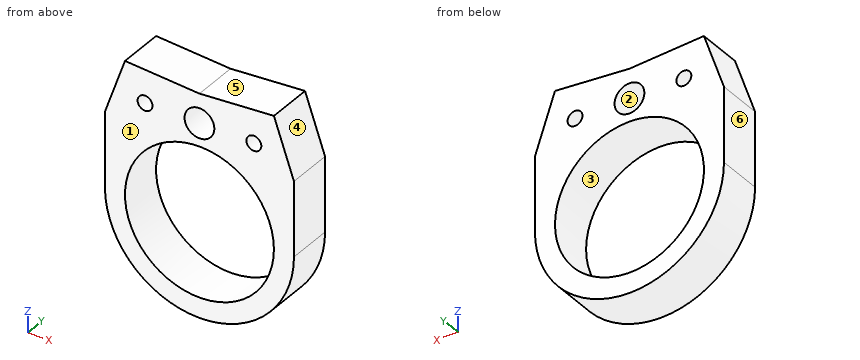
from build123d import *

# Parameters (mm, degrees)
F0_R     = 8.255
F1_DEPTH = 5.08
F3_DEPTH = 5.08
F4_R     = 1.651
F4_R_2   = 0.8255
F5_DEPTH = 25.4


with BuildPart() as f1:
    # F0 (on Front) → F1 (new body)
    with BuildSketch(Plane.XZ):
        with BuildLine():
            ThreePointArc((-10.4775, 0), (0, 10.4775), (10.4775, 0))
            Line((10.4775, 0), (10.4775, 8.255))
            Line((10.4775, 8.255), (6.0325, 10.795))
            Line((6.0325, 10.795), (-6.0325, 10.795))
            Line((-6.0325, 10.795), (-10.4775, 8.255))
            Line((-10.4775, 8.255), (-10.4775, 0))
        make_face()
        with BuildLine():
            ThreePointArc((-10.4775, 0), (0, -10.4775), (10.4775, 0))
            ThreePointArc((10.4775, 0), (0, 10.4775), (-10.4775, 0))
        make_face()
        Circle(F0_R, mode=Mode.SUBTRACT)
    extrude(amount=F1_DEPTH)

    # F2 (on face) → F3 (join)
    with BuildSketch(Plane.XZ.offset(5.08)):
        Polygon((0, 14.0335), (-8.255, 14.605), (-10.4775, 8.255), (-6.0325, 10.795), (6.0325, 10.795), (10.4775, 8.255), (8.255, 14.605), align=None)
    extrude(amount=-F3_DEPTH)

    # F4 (on face) → F5 (cut)
    with BuildSketch(Plane.XZ.offset(5.08)):
        with Locations((0, 10.795)):
            Circle(F4_R)
        with Locations((6.0325, 10.795)):
            Circle(F4_R_2)
        with Locations((-6.0325, 10.795)):
            Circle(F4_R_2)
    extrude(amount=-F5_DEPTH, mode=Mode.SUBTRACT)


solid = f1.part
Work out the finished part from the listing and answer in its coordinate system (mm). Face numbers are marked on the shaded views. A direction names the side the tool comes from. Give positions to 0.01 mm unless a question says otherwise; leave off trailing zeros. Write each loop counter-clockwise with the first axis right and the second up, starting at its lowest first coordinate (ties: lowest second). Pieces come first, ordered by that corner, then holes.
Q1. Given pin 1 (2 mm diameter, centred on y = -1, z = -3, fed in from -X); pin 2 (1.3 mm diameter, centred on x = -6.03, z = 10.8, fed in from -Y); pin 3 (1.5 mm diameter, centred on y = -4, z = -2, fed in from -X), each flat-ended and moving along its own axis, determine where each tip first touches the part or whether it passes through.
Answer:
pin 1: stops at x = -10.28
pin 2: passes through
pin 3: stops at x = -10.4
Q2. The part is cut by section B-B on x = -2. Give the vertices of the cut face in (y, z).
Answer:
outline: (-5.08, -10.28) - (0, -10.28) - (0, -8.01) - (-5.08, -8.01) - close; (-5.08, 8.01) - (0, 8.01) - (0, 14.17) - (-5.08, 14.17) - close
Q3. The part is cut by section A-A on z = -7. Give the vertices of the cut face in (x, y), and give its area (3 significant figures).
Answer:
outline: (-7.8, -5.08) - (-4.38, -5.08) - (-4.38, 0) - (-7.8, 0) - close; (4.38, -5.08) - (7.8, -5.08) - (7.8, 0) - (4.38, 0) - close
area: 34.8 mm2
Q4. Straight lines are drawn through the part: L1, parallel to Z at x = 0, y = -1.9 (1 decimal); L2, parallel to Z at x = -6, y = -1.5; L3, parallel to X at y = -0.25, z = -2.75. For each, find the intervals that lie inside material, in ascending order.
Answer:
L1: z = -10.5 to -8.3, 8.3 to 9.1, 12.4 to 14
L2: z = -8.59 to -5.67, 5.67 to 9.97, 11.62 to 14.45
L3: x = -10.11 to -7.78, 7.78 to 10.11
Q5. For a pull along X with two mould halves and no side action, classify the marked faces 1, 2, 3 and 4 as released by +X, released by -X, zero draft, split by the parting line, or undercut.
Answer:
face 1: zero draft
face 2: undercut
face 3: undercut
face 4: released by +X
Q6. The part is cut by section C-C on y = -2.75. Give the vertices of the cut face in (x, z) (1 decimal).
Answer:
outline: (-10.5, 0) arc R10.5 ccw to (10.5, 0) - (10.5, 8.3) - (8.3, 14.6) - (0, 14) - (-8.3, 14.6) - (-10.5, 8.3) - close; hole circle Ø16.5 at (0, 0); hole circle Ø1.7 at (-6, 10.8); hole circle Ø3.3 at (0, 10.8); hole circle Ø1.7 at (6, 10.8)
Q7. A tool of negligible diameter and unlimited length cuts with its end or side. For the marked faces 5 and 6, from which of +Z, -Z, +X, -X, +Y, -Y can it reach the whole face along a straight path? Write none if from no direction.
Answer:
face 5: +Z, +Y, -Y
face 6: +Z, -Z, -X, +Y, -Y
